Geometry check sheet. Reference: the model listing, model coordinates, mm. Face numbers are marked on the shaded views. A direction names the side the tool comes from. Round coordinates to 2 decimals unless told otherwise and drop trailing zeros. Loops run counter-clockwise (first coordinate to the right, second up) from the corner with the lowest first, then second, coordinate; pieces in that order, holes last. Notation, with made-up numbers: (65, 80) -> (69, 80) arc R17 cw to (69, 99) -> close; hole circle Ø2 at (50, -25). An arc over 180 degrees is marked (long way). Use a Markdown table: item, result. Add a question column.
Q1. Sectioned sample at A-A, the plane z = -2. Enter the section's corners in (x, y).
Q2. Gauge pin test, flat ends, axial feed: P1, Ø5, axis at x = -2, y = 0, coming from the +Z side; P2, Ø3, axis at x = -6.5, y = 2, coming from the -Z side; P3, Ø1.3, axis at x = 12.5, y = -2.5, coming from the -Z side. Record the tip position at first contact, or that the pin passes through.
Q3. Sectioned sample at B-B, the plane z = -5.5. Enter the section's corners in (x, y).
Q4. Set-up check for the marked faces 5, 6, 7 and 8: record each of +Z, -Z, +X, -X, +Y, -Y from which the full face is reachable in a straight line by a thin tool's end or side.
Q5. Release check for a two-part mould opening along Z. For the marked faces 1, 2, 3 and 4 record: released by +Z, released by -Z, zero draft, split by the parting line, or undercut.
Q6. Material ranges on L1, parallel to Y at x = 0, z = -7.8; L2, parallel to X at y = 0, z = 10.7; L3, parallel to Y at x = 0, z = 7.7, recorded low to high.
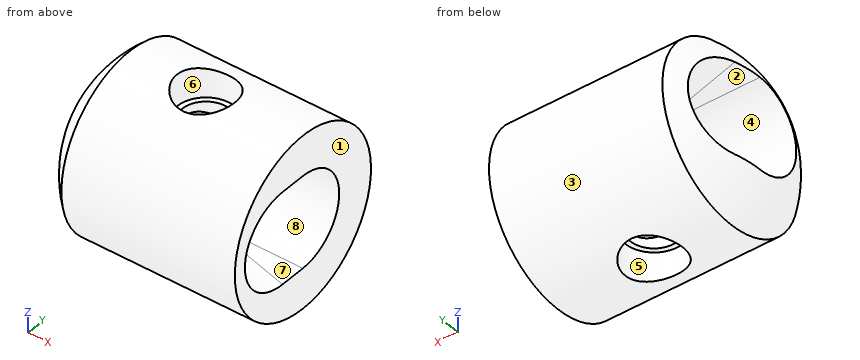
```python
from build123d import *

# Parameters (mm, degrees)
SKIZZE8_R                            = 8
SCHNITT_LINEAR_AUSTRAGEN1_DEPTH      = 21.082062981
SCHNITT_LINEAR_AUSTRAGEN1_DEPTH_BACK = 22.587998658
SCHNITT_LINEAR_AUSTRAGEN2_DEPTH      = 8
SCHNITT_LINEAR_AUSTRAGEN2_DEPTH_BACK = 8


with BuildPart() as part:
    # Skizze4 → Rotation1 (revolve)
    with BuildSketch(Plane(origin=(0, 0, 0), x_dir=(1, 0, 0), z_dir=(0, 1, 0))):
        with BuildLine():
            Line((-13.228756555, 15), (16.771243445, 15))
            Line((16.771243445, 15), (16.771243445, 8))
            Line((16.771243445, 8), (-18.33030278, 8))
            ThreePointArc((-18.33030278, 8), (-16.163030549, 11.779492496), (-13.228756555, 15))
        make_face()
    revolve(axis=Axis((-20, 0, 0), (1, 0, 0)))

    # Skizze6 → Schnitt-Rotation1 (revolve, cut)
    with BuildSketch(Plane(origin=(0, 0, 0), x_dir=(1, 0, 0), z_dir=(0, 1, 0))):
        Polygon((-4.1, 9.5), (-4.1, -9.5), (-5, -9.5), (-5, -15), (0, -15), (0, 15), (-5, 15), (-5, 9.5), align=None)
    revolve(axis=Axis((0, 0, -15), (0, 0, 1)), mode=Mode.SUBTRACT)

    # Skizze8 → Schnitt-Linear austragen1 (cut, two sides)
    with BuildSketch(Plane(origin=(0, 0, 0), x_dir=(0, 0, -1), z_dir=(0.965925826, -0.258819045, 0))) as schnitt_linear_austragen1_sk:
        Circle(SKIZZE8_R)
    extrude(amount=SCHNITT_LINEAR_AUSTRAGEN1_DEPTH, mode=Mode.SUBTRACT)
    extrude(schnitt_linear_austragen1_sk.sketch, amount=-SCHNITT_LINEAR_AUSTRAGEN1_DEPTH_BACK, mode=Mode.SUBTRACT)

    # Skizze9 → Schnitt-Linear austragen2 (cut, two sides)
    with BuildSketch(Plane.XY) as schnitt_linear_austragen2_sk:
        with BuildLine():
            Line((-17.705712859, 4.744231462), (-3.960295888, 1.061158085))
            ThreePointArc((-3.960295888, 1.061158085), (-4.064923932, 0.535157388), (-4.1, 0))
            Line((-4.1, 0), (-18.33030278, 0))
            Line((-18.33030278, 0), (-18.33030278, 2.413230142))
            Line((-18.33030278, 2.413230142), (-17.705712859, 4.744231462))
        make_face()
        with BuildLine():
            Line((16.771243445, -4.493841137), (16.771243445, 0))
            Line((16.771243445, 0), (4.1, 0))
            ThreePointArc((4.1, 0), (4.064923932, -0.535157388), (3.960295888, -1.061158085))
            Line((3.960295888, -1.061158085), (16.771243445, -4.493841137))
        make_face()
    extrude(amount=SCHNITT_LINEAR_AUSTRAGEN2_DEPTH, mode=Mode.SUBTRACT)
    extrude(schnitt_linear_austragen2_sk.sketch, amount=-SCHNITT_LINEAR_AUSTRAGEN2_DEPTH_BACK, mode=Mode.SUBTRACT)


solid = part.part
```
Values:
| question | item | result |
|---|---|---|
| 1 | outline | (-18.33, -7.75) arc R19.9 ccw to (-13.23, -14.87) -> (16.77, -14.87) -> (16.77, -12.51) -> (-1.02, -7.75) -> close; (-15.7, 12.23) -> (1.02, 7.75) -> (16.77, 7.75) -> (16.77, 14.87) -> (-13.23, 14.87) arc R19.9 ccw to start |
| 2 | P1 | z = 9.5 |
| 2 | P2 | z = -14.99 |
| 2 | P3 | z = -14.89 |
| 3 | outline | (-18.33, -5.81) arc R19.23 ccw to (-13.23, -13.96) -> (16.77, -13.96) -> (16.77, -10.51) -> (-0.76, -5.81) -> close; (-16.2, 10.36) -> (0.76, 5.81) -> (16.77, 5.81) -> (16.77, 13.96) -> (-13.23, 13.96) arc R19.23 ccw to start |
| 4 | face 5 | -Z |
| 4 | face 6 | +Z |
| 4 | face 7 | +X |
| 4 | face 8 | +X, -X |
| 5 | face 1 | zero draft |
| 5 | face 2 | undercut |
| 5 | face 3 | split by the parting line |
| 5 | face 4 | undercut |
| 6 | L1 | -12.81 to -4.1, 4.1 to 12.81 |
| 6 | L2 | -16.9 to -5, 5 to 16.77 |
| 6 | L3 | -12.87 to -4.1, 4.1 to 12.87 |
